For this review, use the dimensioned drawing (mm, ordinates from the lowest corner) and the shaded views. Give positions to 0.01 mm unless a question says otherwise; leave off trailing zeros. Order: outer loops, then holes, each group sorted by start corner. A loop starts at its lowest first (then second) coordinate and runs counter-clockwise, first axis right, second up. Notation, with made-up numbers: (40, 39) -> (69, 39) arc R8 ccw to (69, 52) -> close; hole circle Ø8 at (31, 20.25). An arc over 180 degrees is marked (long way). Return JSON: item names as keys, results as strings.
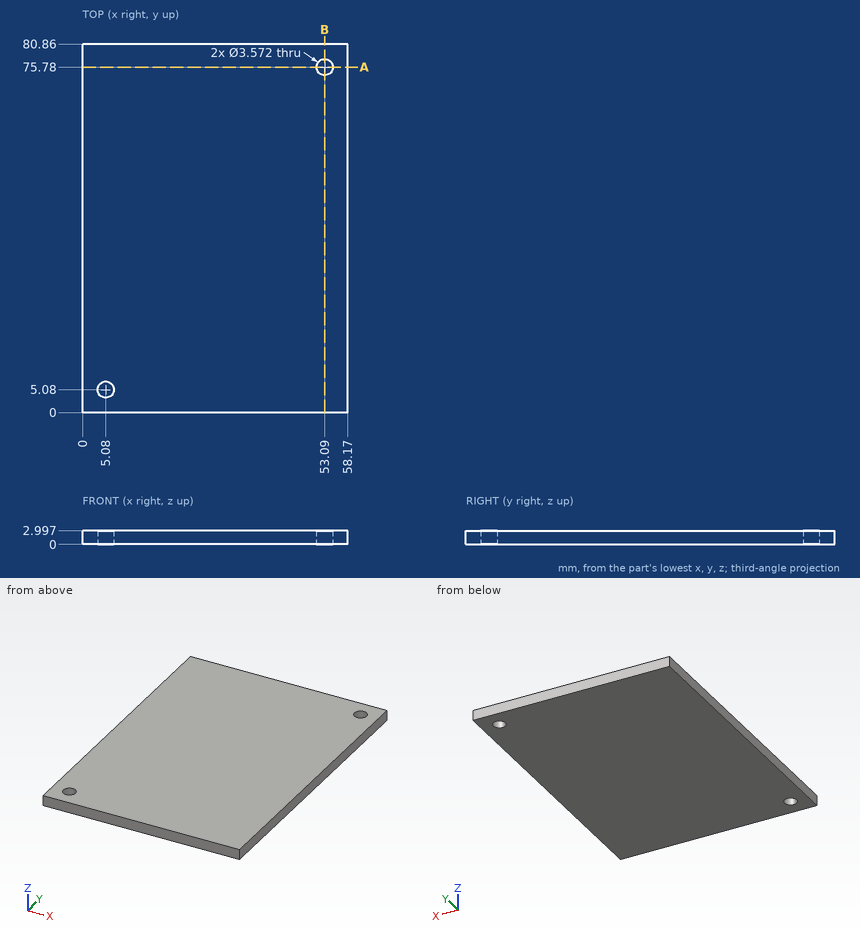
Item 1: Add section A-A (y = 75.78). Give the boundary of the cut face in (x, z).
Result set:
{"outline": "(0, 0) -> (51.3, 0) -> (51.3, 3) -> (0, 3) -> close; (54.88, 0) -> (58.17, 0) -> (58.17, 3) -> (54.88, 3) -> close"}
Item 2: Wall thickness on L1, parallel to Y at x = 53.09, z = 2.3; L2, parallel to Y at x = 5.08, z = 2.25: over which ranges is each line inside the solid? List them lowest first. Write a range as [from, to].
Result set:
{"L1": "y = [0, 73.99], [77.57, 80.86]", "L2": "y = [0, 3.29], [6.87, 80.86]"}
Item 3: For pin 1 (2 mm diameter, centred on x = 5.08, y = 5.08, fed in from -Z) (1 decimal), flat-tipped, find the tip position at first contact; note if it passes through.
Result set:
{"pin 1": "passes through"}
Item 4: Add section B-B (x = 53.09). Give the boundary of the cut face in (y, z).
Result set:
{"outline": "(0, 0) -> (73.99, 0) -> (73.99, 3) -> (0, 3) -> close; (77.57, 0) -> (80.86, 0) -> (80.86, 3) -> (77.57, 3) -> close"}
